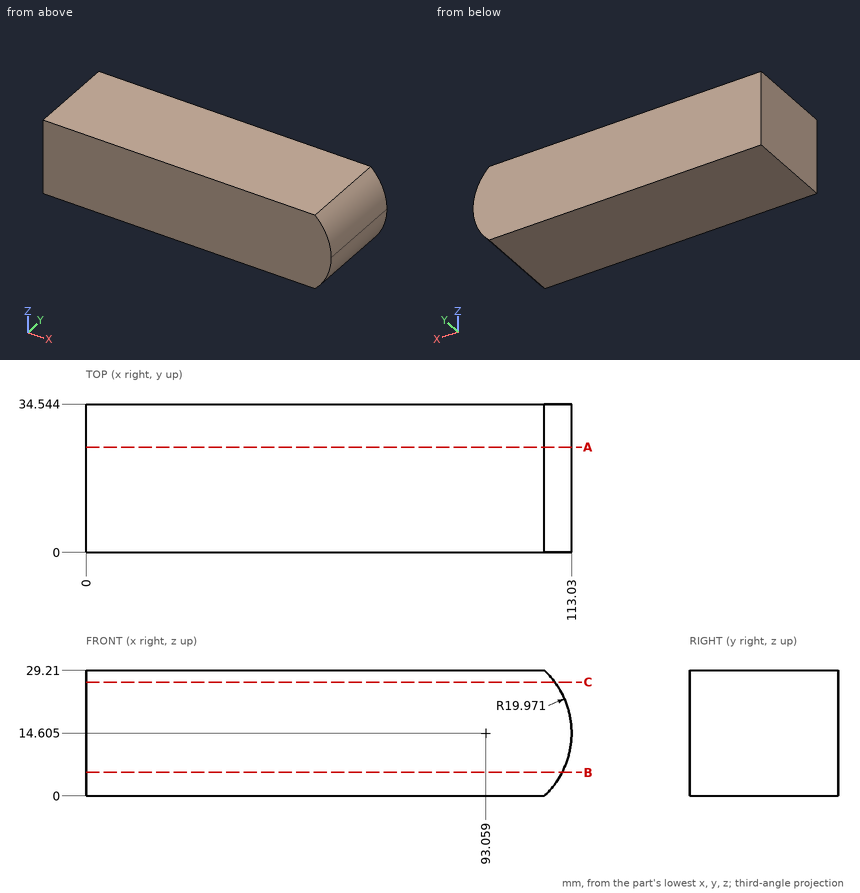
Print and shaded views of the part. All mm, measured from the part's lowest x, y and z. Coordinates: 2 decimals unless noted, no trailing zeros. Order: outer loops, then holes, each group sorted by start corner. A loop starts at its lowest first (then second) coordinate and runs counter-clockwise, first axis right, second up.
(1) Slice it at C-C, the plane z = 26.5. Write the cut outline in (x, y).
Check sheet entries:
outline: (0, 0) - (109.1, 0) - (109.1, 34.54) - (0, 34.54) - close
(2) Slice it at A-A, the plane y = 24.5. Write the cut outline in (x, z) (1 decimal).
Check sheet entries:
outline: (0, 0) - (106.7, 0) arc R20 ccw to (106.7, 29.2) - (0, 29.2) - close
(3) Probe L1, parallel to X at y = 15, z = 15; L2, parallel to X at y = 14, z = 3.75; L3, parallel to Z at x = 107, y = 28 (1 decimal). List the from-to ranges inside material, lowest first.
Check sheet entries:
L1: x = 0 to 113.03
L2: x = 0 to 109.82
L3: z = 0.3 to 28.9
(4) Slice it at B-B, the plane z = 5.5. Write the cut outline in (x, y).
Check sheet entries:
outline: (0, 0) - (110.83, 0) - (110.83, 34.54) - (0, 34.54) - close
(5) Pin check, flat tips, straight feed: pin 1 Ø3 at (y, z) = (19, 9.5) entering from +X; pin 2 Ø1 at (y, z) = (29, 13) entering from +X. Stop position of each tip, or through.
Check sheet entries:
pin 1: stops at x = 112.7
pin 2: stops at x = 113
